Here's how the part is built. I have some questions about the finished solid (model axes, mm). Face numbers are marked on the shaded views. A direction names the side the tool comes from. Coordinates: 2 decimals unless noted, no trailing zeros. Write each loop counter-clockwise with the first axis right and the second up, starting at its lowest first coordinate (ties: lowest second). Pieces come first, ordered by that corner, then holes.
(1) Imagine slicing it at B-B, the plane y = 15. State how many separate pieces and enclosed holes the cut face has, plus the area to 3 significant figures.
(2) Which directions (+Z, -Z, +X, -X, +Y, -Y) give clear straight access to the entire face, cutting with the end or side of a thin tool? Please do the marked faces 5, 6, 7 and 8.
(3) Please list where these lines run through material, in increasing order: probe 1 along Y at (x, z) = (16, 3.05); probe 2 along Z at (x, y) = (14, -22); probe 3 along Y at (x, z) = (6.5, 110).
(4) Thinking about a two-plate mould opening in Z: for the marked faces 1, 2, 3 and 4, which applies, released by +Z, released by -Z, zero draft, split by the parting line, or undercut?
(5) For pin 1 Ø5 at (y, z) = (-6, 172.5) entering from -X; pin 2 Ø4.5 at (y, z) = (3.5, 2.5) entering from -X; pin 3 Ø4 at (x, y) = (-19, -15) entering from -Z, each with a flat end and sliding along its axis, tell me the tip position at first contact or that it passes through.
(6) Imagine slicing it at C-C, the plane z = 16.5. List the corners of the cut face in (x, y) for me, plus the area to 3 significant figures.
```python
from build123d import *

# Parameters (mm, degrees)
EXTRUDE_1_DEPTH     = 150
FILLET_1_R          = 5
SKETCH_2_W          = 47
SKETCH_2_H          = 45
SKETCH_2_R          = 2.15
EXTRUDE_2_DEPTH     = 4
EXTRUDE_START       = 74
SKETCH_3_W          = 20.5
SKETCH_3_H          = 40
EXTRUDE_3_DEPTH     = 3
EXTRUDE_START_2     = 147
SKETCH_4_W          = 20.5
SKETCH_4_H          = 40
EXTRUDE_4_DEPTH     = 3
EXTRUDE_START_3     = 104
EXTRUDE_5_DEPTH     = 4
EXTRUDE_START_4     = 108
EXTRUDE_6_DEPTH     = 50
EXTRUDE_START_5     = 158
EXTRUDE_7_DEPTH     = 4
EXTRUDE_START_6     = 162
EXTRUDE_8_DEPTH     = 66
EXTRUDE_START_7     = 228
EXTRUDE_9_DEPTH     = 4
FILLET_2_R          = 8
FILLET_3_R          = 6
FILLET_4_R          = 5
FILLET_5_R          = 5
FILLET_6_R          = 5
CUT_EXTRUDE_START   = 77
SKETCH_10_W         = 49
SKETCH_10_H         = 39
CUT_EXTRUDE_1_DEPTH = 70
CUT_EXTRUDE_START_2 = 157
CUT_EXTRUDE_2_DEPTH = 8
CUT_EXTRUDE_START_3 = 166
SKETCH_12_W         = 11
SKETCH_12_H         = 40
CUT_EXTRUDE_3_DEPTH = 58


with BuildPart() as part:
    # 草圖1 → 填料-伸長1 (new body)
    with BuildSketch(Plane.XY):
        Polygon((-13, -22.5), (10, -22.5), (10, -19.5), (-10, -19.5), (-10, 19.5), (10, 19.5), (10, 22.5), (-13, 22.5), align=None)
    extrude(amount=EXTRUDE_1_DEPTH)

    # 圓角1
    fillet_1_edges = [part.edges().sort_by_distance(p)[0] for p in [
        (-13, 22.5, 75),
        (-13, -22.5, 75),
    ]]
    fillet(fillet_1_edges, radius=FILLET_1_R)

    # 草圖2 → 填料-伸長2 (add)
    with BuildSketch(Plane.XY):
        with Locations((-1.5, 0)):
            Rectangle(SKETCH_2_W, SKETCH_2_H)
        with Locations((-19, 15)):
            Circle(SKETCH_2_R, mode=Mode.SUBTRACT)
        with Locations((-19, -15)):
            Circle(SKETCH_2_R, mode=Mode.SUBTRACT)
        with Locations((16, 15)):
            Circle(SKETCH_2_R, mode=Mode.SUBTRACT)
        with Locations((16, -15)):
            Circle(SKETCH_2_R, mode=Mode.SUBTRACT)
    extrude(amount=EXTRUDE_2_DEPTH)

    # 草圖3 → 填料-伸長3 (add)
    with BuildSketch(Plane.XY.offset(EXTRUDE_START)):
        with Locations((-0.25, 0)):
            Rectangle(SKETCH_3_W, SKETCH_3_H)
    extrude(amount=EXTRUDE_3_DEPTH)

    # 草圖4 → 填料-伸長4 (add)
    with BuildSketch(Plane.XY.offset(EXTRUDE_START_2)):
        with Locations((-0.25, 0)):
            Rectangle(SKETCH_4_W, SKETCH_4_H)
    extrude(amount=EXTRUDE_4_DEPTH)

    # 草圖5 → 填料-伸長5 (add)
    with BuildSketch(Plane.XY.offset(EXTRUDE_START_3)):
        with BuildLine():
            Line((34, -32), (34, 32))
            ThreePointArc((34, 32), (30.485281374, 40.485281374), (22, 44))
            Line((22, 44), (-22, 44))
            ThreePointArc((-22, 44), (-30.485281374, 40.485281374), (-34, 32))
            Line((-34, 32), (-34, -32))
            ThreePointArc((-34, -32), (-30.485281374, -40.485281374), (-22, -44))
            Line((-22, -44), (22, -44))
            ThreePointArc((22, -44), (30.485281374, -40.485281374), (34, -32))
        make_face()
    extrude(amount=EXTRUDE_5_DEPTH)

    # 草圖6 → 填料-伸長6 (add)
    with BuildSketch(Plane.XY.offset(EXTRUDE_START_4)):
        with BuildLine():
            Line((34, -32), (34, 32))
            ThreePointArc((34, 32), (30.485281374, 40.485281374), (22, 44))
            Line((22, 44), (-22, 44))
            ThreePointArc((-22, 44), (-30.485281374, 40.485281374), (-34, 32))
            Line((-34, 32), (-34, -32))
            ThreePointArc((-34, -32), (-30.485281374, -40.485281374), (-22, -44))
            Line((-22, -44), (22, -44))
            ThreePointArc((22, -44), (30.485281374, -40.485281374), (34, -32))
        make_face()
        with BuildLine():
            Line((30, -32), (30, 32))
            ThreePointArc((30, 32), (27.656854249, 37.656854249), (22, 40))
            Line((22, 40), (-22, 40))
            ThreePointArc((-22, 40), (-27.656854249, 37.656854249), (-30, 32))
            Line((-30, 32), (-30, -32))
            ThreePointArc((-30, -32), (-27.656854249, -37.656854249), (-22, -40))
            Line((-22, -40), (22, -40))
            ThreePointArc((22, -40), (27.656854249, -37.656854249), (30, -32))
        make_face(mode=Mode.SUBTRACT)
    extrude(amount=EXTRUDE_6_DEPTH)

    # 草圖7 → 填料-伸長7 (add)
    with BuildSketch(Plane.XY.offset(EXTRUDE_START_5)):
        with BuildLine():
            Line((34, -32), (34, 32))
            ThreePointArc((34, 32), (30.485281374, 40.485281374), (22, 44))
            Line((22, 44), (-22, 44))
            ThreePointArc((-22, 44), (-30.485281374, 40.485281374), (-34, 32))
            Line((-34, 32), (-34, -32))
            ThreePointArc((-34, -32), (-30.485281374, -40.485281374), (-22, -44))
            Line((-22, -44), (22, -44))
            ThreePointArc((22, -44), (30.485281374, -40.485281374), (34, -32))
        make_face()
    extrude(amount=EXTRUDE_7_DEPTH)

    # 草圖8 → 填料-伸長8 (add)
    with BuildSketch(Plane.XY.offset(EXTRUDE_START_6)):
        with BuildLine():
            Line((23.5, -23.5), (23.5, 23.5))
            ThreePointArc((23.5, 23.5), (20.571067812, 30.571067812), (13.5, 33.5))
            Line((13.5, 33.5), (-13.5, 33.5))
            ThreePointArc((-13.5, 33.5), (-20.571067812, 30.571067812), (-23.5, 23.5))
            Line((-23.5, 23.5), (-23.5, -23.5))
            ThreePointArc((-23.5, -23.5), (-20.571067812, -30.571067812), (-13.5, -33.5))
            Line((-13.5, -33.5), (13.5, -33.5))
            ThreePointArc((13.5, -33.5), (20.571067812, -30.571067812), (23.5, -23.5))
        make_face()
        with BuildLine():
            Line((19.5, -23.5), (19.5, 23.5))
            ThreePointArc((19.5, 23.5), (17.742640687, 27.742640687), (13.5, 29.5))
            Line((13.5, 29.5), (-13.5, 29.5))
            ThreePointArc((-13.5, 29.5), (-17.742640687, 27.742640687), (-19.5, 23.5))
            Line((-19.5, 23.5), (-19.5, -23.5))
            ThreePointArc((-19.5, -23.5), (-17.742640687, -27.742640687), (-13.5, -29.5))
            Line((-13.5, -29.5), (13.5, -29.5))
            ThreePointArc((13.5, -29.5), (17.742640687, -27.742640687), (19.5, -23.5))
        make_face(mode=Mode.SUBTRACT)
    extrude(amount=EXTRUDE_8_DEPTH)

    # 草圖9 → 填料-伸長9 (add)
    with BuildSketch(Plane.XY.offset(EXTRUDE_START_7)):
        with BuildLine():
            Line((23.5, -23.5), (23.5, 23.5))
            ThreePointArc((23.5, 23.5), (20.571067812, 30.571067812), (13.5, 33.5))
            Line((13.5, 33.5), (-13.5, 33.5))
            ThreePointArc((-13.5, 33.5), (-20.571067812, 30.571067812), (-23.5, 23.5))
            Line((-23.5, 23.5), (-23.5, -23.5))
            ThreePointArc((-23.5, -23.5), (-20.571067812, -30.571067812), (-13.5, -33.5))
            Line((-13.5, -33.5), (13.5, -33.5))
            ThreePointArc((13.5, -33.5), (20.571067812, -30.571067812), (23.5, -23.5))
        make_face()
    extrude(amount=EXTRUDE_9_DEPTH)

    # 圓角2
    fillet_2_edges = [part.edges().sort_by_distance(p)[0] for p in [
        (-11.535533906, -21.035533906, 104),
        (1, 22.5, 104),
        (-13, 0, 104),
        (1, -22.5, 104),
        (-11.535533906, 21.035533906, 104),
    ]]
    fillet(fillet_2_edges, radius=FILLET_2_R)

    # 圓角3
    fillet_3_edges = [part.edges().sort_by_distance(p)[0] for p in [
        (30.485281374, -40.485281374, 104),
        (34, 0, 104),
        (30.485281374, 40.485281374, 104),
        (0, 44, 104),
        (-30.485281374, 40.485281374, 104),
        (-34, 0, 104),
        (-30.485281374, -40.485281374, 104),
        (0, -44, 104),
    ]]
    fillet(fillet_3_edges, radius=FILLET_3_R)

    # 圓角4
    fillet_4_edges = [part.edges().sort_by_distance(p)[0] for p in [
        (30.485281374, -40.485281374, 162),
        (34, 0, 162),
        (30.485281374, 40.485281374, 162),
        (0, 44, 162),
        (-30.485281374, 40.485281374, 162),
        (-34, 0, 162),
        (-30.485281374, -40.485281374, 162),
        (0, -44, 162),
    ]]
    fillet(fillet_4_edges, radius=FILLET_4_R)

    # 圓角5
    fillet_5_edges = [part.edges().sort_by_distance(p)[0] for p in [
        (20.571067812, -30.571067812, 162),
        (23.5, 0, 162),
        (20.571067812, 30.571067812, 162),
        (0, 33.5, 162),
        (-20.571067812, 30.571067812, 162),
        (-23.5, 0, 162),
        (-20.571067812, -30.571067812, 162),
        (0, -33.5, 162),
    ]]
    fillet(fillet_5_edges, radius=FILLET_5_R)

    # 圓角6
    fillet_6_edges = [part.edges().sort_by_distance(p)[0] for p in [
        (20.571067812, -30.571067812, 232),
        (23.5, 0, 232),
        (20.571067812, 30.571067812, 232),
        (0, 33.5, 232),
        (-20.571067812, 30.571067812, 232),
        (-23.5, 0, 232),
        (-20.571067812, -30.571067812, 232),
        (0, -33.5, 232),
    ]]
    fillet(fillet_6_edges, radius=FILLET_6_R)

    # 草圖10 → 除料-伸長1 (cut)
    with BuildSketch(Plane.XY.offset(CUT_EXTRUDE_START)):
        with Locations((14.5, 0)):
            Rectangle(SKETCH_10_W, SKETCH_10_H)
    extrude(amount=CUT_EXTRUDE_1_DEPTH, mode=Mode.SUBTRACT)

    # 草圖11 → 除料-伸長2 (cut)
    with BuildSketch(Plane.XY.offset(CUT_EXTRUDE_START_2)):
        with BuildLine():
            Line((19.5, -23.5), (19.5, 23.5))
            ThreePointArc((19.5, 23.5), (17.742640687, 27.742640687), (13.5, 29.5))
            Line((13.5, 29.5), (-13.5, 29.5))
            ThreePointArc((-13.5, 29.5), (-17.742640687, 27.742640687), (-19.5, 23.5))
            Line((-19.5, 23.5), (-19.5, -23.5))
            ThreePointArc((-19.5, -23.5), (-17.742640687, -27.742640687), (-13.5, -29.5))
            Line((-13.5, -29.5), (13.5, -29.5))
            ThreePointArc((13.5, -29.5), (17.742640687, -27.742640687), (19.5, -23.5))
        make_face()
    extrude(amount=CUT_EXTRUDE_2_DEPTH, mode=Mode.SUBTRACT)

    # 草圖12 → 除料-伸長3 (cut)
    with BuildSketch(Plane.XY.offset(CUT_EXTRUDE_START_3)):
        with Locations((23, 0)):
            Rectangle(SKETCH_12_W, SKETCH_12_H)
    extrude(amount=CUT_EXTRUDE_3_DEPTH, mode=Mode.SUBTRACT)


solid = part.part
```
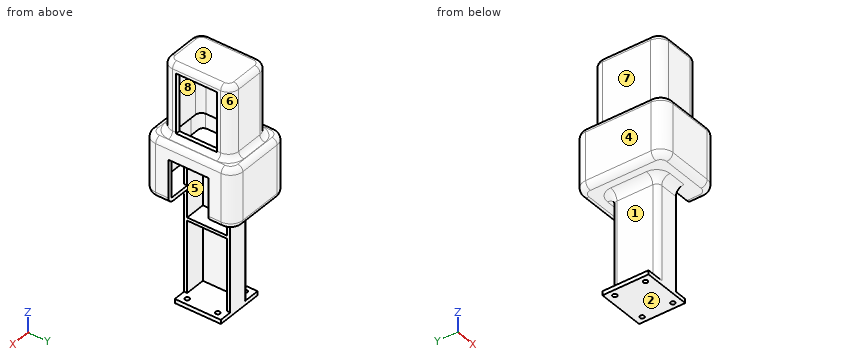
Recorded:
1. separate pieces: 4
1. enclosed holes: 0
1. area: 1,630 mm2
2. face 5: +X
2. face 6: +Z, +X, +Y
2. face 7: +Z, -X, +Y, -Y
2. face 8: none
3. probe 1: y = -22.5 to -17.15, -12.85 to 12.85, 17.15 to 22.5
3. probe 2: z = 0 to 4, 104 to 108, 228 to 232
3. probe 3: y = -44 to -40, -22.5 to -19.5, 19.5 to 22.5, 40 to 44
4. face 1: undercut
4. face 2: released by -Z
4. face 3: released by +Z
4. face 4: zero draft
5. pin 1: stops at x = -23.5
5. pin 2: stops at x = -25
5. pin 3: stops at z = 102.93
6. outline: (-13, -17.5) arc R5 ccw to (-8, -22.5) - (10, -22.5) - (10, -19.5) - (-10, -19.5) - (-10, 19.5) - (10, 19.5) - (10, 22.5) - (-8, 22.5) arc R5 ccw to (-13, 17.5) - close
6. area: 244 mm2
